The listing builds one solid part. Answer for the finished solid, in the listing's coordinates (mm). A direction names the side the tool comes from. Round coordinates to 2 decimals unless told otherwise and drop trailing zeros. Order: outer loops, then holes, each group sorted by start corner. A loop starts at its lowest first (then second) coordinate and runs counter-clockwise, first axis right, second up. Notation, with made-up numbers: M 62,66.5 L 110,66.5 A17 cw 110,94.5 Z; hole C 48,81.5 d3. An arc over 180 degrees is marked long. Write item = value, one per line. Start each with the question number.
(1) Straight lines are drawn through the part: probe 1 along Z at (x, y) = (87.25, 1.25); probe 2 along X at (y, z) = (1.2, -10); probe 3 along X at (y, z) = (4.3, -10). For each, find the intervals that lie inside material, in ascending order. Write a range as from..to.
(2) A cutting plane is placed at A-A, the plane x = -87.25. Determine the outline of the cut face in (y, z), and give its area (3 significant figures).
(3) Which of the six approach directions +Z, -Z, +X, -X, +Y, -Y give full straight-line access (tool end or side, diameter ignored) to faces 1 (the face through (-89.233, 2.662, -9.74)), 2 (the face through (-37, 3.7, 51))?
(4) This flat-tipped pin is pushed along its axis until it touches: pin 1 (2.5 mm diameter, centred on x = -87.25, z = -10, fed in from +Y). Where does it stop, or does it pass through?
(5) For a pull along X with two mould halves and no side action, classify faces 3 (the face through (0, 0, -55)), 4 (the face through (13.846, 2.662, -56.503)), 5 (the face through (91.25, 3, -2)) as released by +X, released by -X, zero draft, split by the parting line, or undercut.
(6) A cutting plane is placed at C-C, the plane y = 2.75. Determine the outline of the cut face in (x, z).
(7) A cutting plane is placed at D-D, the plane z = -60. Determine the outline of the cut face in (x, y).
(8) A cutting plane is placed at B-B, the plane z = -18. Determine the outline of the cut face in (x, y).
from build123d import *

# Parameters (mm, degrees)
SKETCH1_W               = 182.5
SKETCH1_H               = 128
SKETCH1_R               = 3.5
SKETCH1_R_2             = 2
BOSS_EXTRUDE1_DEPTH     = 5.4
CUT_EXTRUDE3_DEPTH      = 114.334560042
CUT_EXTRUDE3_DEPTH_BACK = 114.334560042
SKETCH1_4_W             = 160.5
SKETCH1_4_H             = 101
SKETCH1_5_W             = 3
SKETCH1_5_H             = 101
CUT_EXTRUDE4_DEPTH      = 3.7


with BuildPart() as part:
    # Sketch1 → Boss-Extrude1 (new body)
    with BuildSketch(Plane(origin=(0, 0, 0), x_dir=(1, 0, 0), z_dir=(0, 1, 0))):
        with Locations((0, 3)):
            Rectangle(SKETCH1_W, SKETCH1_H)
        with Locations(Location((-14, 60, 0), (0, 0, 90))):
            Circle(SKETCH1_R, mode=Mode.SUBTRACT)
        with Locations(Location((14, 60, 0), (0, 0, 90))):
            Circle(SKETCH1_R, mode=Mode.SUBTRACT)
        with Locations(Location((-87.25, -10, 0), (0, 0, 90))):
            Circle(SKETCH1_R_2, mode=Mode.SUBTRACT)
        with Locations(Location((87.25, -10, 0), (0, 0, 90))):
            Circle(SKETCH1_R_2, mode=Mode.SUBTRACT)
        with Locations(Location((-87.25, 10, 0), (0, 0, 90))):
            Circle(SKETCH1_R_2, mode=Mode.SUBTRACT)
        with Locations(Location((87.25, 10, 0), (0, 0, 90))):
            Circle(SKETCH1_R_2, mode=Mode.SUBTRACT)
    extrude(amount=BOSS_EXTRUDE1_DEPTH)

    # Sketch1_4 → Cut-Extrude3 (cut, two sides: drawn at the far end of the back side and taken through both)
    with BuildSketch(Plane(origin=(0, 0, 0), x_dir=(1, 0, 0), z_dir=(0, 1, 0)).offset(-CUT_EXTRUDE3_DEPTH_BACK)):
        with Locations((0, 2.5)):
            Rectangle(SKETCH1_4_W, SKETCH1_4_H)
    extrude(amount=CUT_EXTRUDE3_DEPTH + CUT_EXTRUDE3_DEPTH_BACK, mode=Mode.SUBTRACT)

    # Sketch1_5 → Cut-Extrude4 (cut)
    with BuildSketch(Plane(origin=(0, 0, 0), x_dir=(1, 0, 0), z_dir=(0, 1, 0))):
        Polygon((-83.25, -48), (-83.25, -53), (83.25, -53), (83.25, -48), (80.25, -48), (-80.25, -48), align=None)
        with Locations((-81.75, 2.5)):
            Rectangle(SKETCH1_5_W, SKETCH1_5_H)
        with Locations((81.75, 2.5)):
            Rectangle(SKETCH1_5_W, SKETCH1_5_H)
    extrude(amount=CUT_EXTRUDE4_DEPTH, mode=Mode.SUBTRACT)


solid = part.part
Reported:
q1.probe_1 = -67..-12, -8..8, 12..61
q1.probe_2 = -91.25..-89.25, -85.25..-83.25, 83.25..85.25, 89.25..91.25
q1.probe_3 = -91.25..-89.25, -85.25..-80.25, 80.25..85.25, 89.25..91.25
q2.outline = M 0,-67 L 5.4,-67 L 5.4,-12 L 0,-12 Z; M 0,-8 L 5.4,-8 L 5.4,8 L 0,8 Z; M 0,12 L 5.4,12 L 5.4,61 L 0,61 Z
q2.area = 648 mm²
q3.face_1 = +Y, -Y
q3.face_2 = -Y
q4.pin_1 = through
q5.face_3 = zero draft
q5.face_4 = undercut
q5.face_5 = released by +X
q6.outline = M -91.25,-67 L 91.25,-67 L 91.25,61 L -91.25,61 Z; hole C -87.25,-10 d4; hole C -87.25,10 d4; hole M -83.25,-53 L 83.25,-53 L 83.25,53 L -83.25,53 Z; hole C -14,-60 d7; hole C 14,-60 d7; hole C 87.25,-10 d4; hole C 87.25,10 d4
q7.outline = M -91.25,0 L -17.5,0 L -17.5,5.4 L -91.25,5.4 Z; M -10.5,0 L 10.5,0 L 10.5,5.4 L -10.5,5.4 Z; M 17.5,0 L 91.25,0 L 91.25,5.4 L 17.5,5.4 Z
q8.outline = M -91.25,0 L -83.25,0 L -83.25,3.7 L -80.25,3.7 L -80.25,5.4 L -91.25,5.4 Z; M 80.25,3.7 L 83.25,3.7 L 83.25,0 L 91.25,0 L 91.25,5.4 L 80.25,5.4 Z
